Work out the finished part from the listing and answer in its coordinate system (mm). A direction names the side the tool comes from. Give positions to 0.01 mm unless a question says otherwise; leave off trailing zeros. Loops run counter-clockwise (first coordinate to the right, second up) from the corner with the lowest first, then second, coordinate; pieces in that order, holes last. Notation, with made-up numbers: M -33,-26.75 L 6,-26.75 A38 ccw 6,11.25 Z; hole C -2.5,-23 d9. An arc over 180 degrees is marked long. Write item = value, one per line. Start each with the question number.
1. Flat-ended cylindrical pins translate along their axes: pin 1 Ø2.5 at (x, y) = (-20.5, 6) entering from -Z; pin 2 Ø1.5 at (x, z) = (6, -4.5) entering from +Y; pin 3 Ø4 at (y, z) = (6.5, -16.5) entering from -X. Find the tip coordinate at first contact, or state that the pin passes through.
2. Section B-B on y = 6 is taken. Give the number of separate pieces and of enclosed holes in the cut face, plus the area to 3 significant figures.
3. For faces 1 (the face through (-21.89, 4.94, 20.07)), 2 (the face through (14, 8, -18)), 3 (the face through (24, 3, 6)), determine the directions among +Z, -Z, +X, -X, +Y, -Y from which every point of the face is accessible in a straight line to the end or side of a thin tool.
4. Section D-D on y = 1 is taken. Determine the outline of the cut face in (x, z), plus the area to 3 significant figures.
5. Consider L1, parallel to X at y = 2.4, z = -8.5; L2, parallel to X at y = 1.8, z = 9; L3, parallel to Y at x = -19.75, z = -17.5. Determine where each line is inside the solid, lowest interval first. Write a range as [from, to].
6. Section A-A on x = -20.5 is taken. Determine the outline of the cut face in (y, z), plus the area to 3 significant figures.
7. Section C-C on z = -17.5 is taken. Determine the outline of the cut face in (x, y), plus the area to 3 significant figures.
8. The mould has two halves that part along Z. Classify faces 4 (the face through (13.57, 2.03, -9.15)), 5 (the face through (-19.43, 2.03, -9.15)), 6 (the face through (-19, 6, -20.5)), 7 (the face through (-26, 2, 0)): released by +Z, released by -Z, zero draft, split by the parting line, or undercut.
```python
from build123d import *

# Parameters (mm, degrees)
SKETCH1_W               = 53
SKETCH1_H               = 55
TOP_DEPTH               = 2
SKETCH2_W               = 48
SKETCH2_H               = 50
INSIDE_LIP_DEPTH        = 2
SKETCH3_W               = 7
SKETCH3_H               = 10
SKETCH3_W_2             = 10
SKETCH3_H_2             = 6
SCREW_POSTS_DEPTH       = 5
SKETCH4_R               = 1.75
FRONT_SCREW_HOLES_DEPTH = 10
BACK_START              = -48
SKETCH5_R               = 1.6
BACK_SCREW_HOLES_DEPTH  = 48
SKETCH6_R               = 3
CUT_EXTRUDE3_DEPTH      = 4


with BuildPart() as part:
    # Sketch1 → Top (new body)
    with BuildSketch(Plane(origin=(0, 0, 0), x_dir=(1, 0, 0), z_dir=(0, 1, 0))):
        Rectangle(SKETCH1_W, SKETCH1_H)
    extrude(amount=TOP_DEPTH)

    # Sketch2 → Inside Lip (add)
    with BuildSketch(Plane(origin=(0, 2, 0), x_dir=(1, 0, 0), z_dir=(0, 1, 0))):
        Rectangle(SKETCH2_W, SKETCH2_H)
    extrude(amount=INSIDE_LIP_DEPTH)

    # Sketch3 → Screw Posts (add)
    with BuildSketch(Plane(origin=(0, 4, 0), x_dir=(1, 0, 0), z_dir=(0, 1, 0))):
        with Locations((-20.5, -20)):
            Rectangle(SKETCH3_W, SKETCH3_H)
        with Locations((20.5, -20)):
            Rectangle(SKETCH3_W, SKETCH3_H)
        with Locations((19, 17.5)):
            Rectangle(SKETCH3_W_2, SKETCH3_H_2)
        with Locations((-19, 17.5)):
            Rectangle(SKETCH3_W_2, SKETCH3_H_2)
    extrude(amount=SCREW_POSTS_DEPTH)

    # Sketch4 → Front Screw Holes (cut)
    with BuildSketch(Plane.XY.offset(25)):
        with Locations((-20.5, 6)):
            Circle(SKETCH4_R)
        with Locations((20.5, 6)):
            Circle(SKETCH4_R)
    extrude(amount=-FRONT_SCREW_HOLES_DEPTH, mode=Mode.SUBTRACT)

    # Sketch5 → Back Screw Holes (cut)
    with BuildSketch(Plane(origin=(24, 0, 0), x_dir=(0, 0, -1), z_dir=(1, 0, 0)).offset(BACK_START)):
        with Locations((17.5, 6)):
            Circle(SKETCH5_R)
    extrude(amount=BACK_SCREW_HOLES_DEPTH, mode=Mode.SUBTRACT)

    # Sketch6 → Cut-Extrude3 (cut)
    with BuildSketch(Plane(origin=(0, 4, 0), x_dir=(1, 0, 0), z_dir=(0, 1, 0))):
        with Locations(Location((-16.5, -9, 0), (0, 0, 270))):
            Circle(SKETCH6_R)
        with Locations(Location((-16.5, 8.5, 0), (0, 0, 270))):
            Circle(SKETCH6_R)
        with Locations(Location((16.5, -9, 0), (0, 0, 270))):
            Circle(SKETCH6_R)
        with Locations(Location((16.5, 8.5, 0), (0, 0, 270))):
            Circle(SKETCH6_R)
    extrude(amount=-CUT_EXTRUDE3_DEPTH, mode=Mode.SUBTRACT)


solid = part.part
```
Verdict:
q1.pin_1 = -20.5
q1.pin_2 = 4
q1.pin_3 = -24
q2.separate_pieces = 8
q2.enclosed_holes = 0
q2.area = 126 mm2
q3.face_1 = +Z
q3.face_2 = +Z, -Z, +Y
q3.face_3 = +Z, -Z, +X, +Y
q4.outline = M -26.5,-27.5 L 26.5,-27.5 L 26.5,27.5 L -26.5,27.5 Z; hole C -16.5,-8.5 d6; hole C -16.5,9 d6; hole C 16.5,-8.5 d6; hole C 16.5,9 d6
q4.area = 2,800 mm2
q5.L1 = [-24, -19.5], [-13.5, 13.5], [19.5, 24]
q5.L2 = [-26.5, -19.5], [-13.5, 13.5], [19.5, 26.5]
q5.L3 = [0, 4.4], [7.6, 9]
q6.outline = M 0,-27.5 L 2,-27.5 L 2,-25 L 4,-25 L 4,-20.5 L 9,-20.5 L 9,-14.5 L 4,-14.5 L 4,15 L 4.25,15 L 4.25,25 L 2,25 L 2,27.5 L 0,27.5 Z; M 7.75,15 L 9,15 L 9,25 L 7.75,25 Z; hole C 6,-17.5 d3.2
q6.area = 247 mm2
q7.outline = M -26.5,0 L 26.5,0 L 26.5,2 L 24,2 L 24,4.4 L 14,4.4 L 14,4 L -14,4 L -14,4.4 L -24,4.4 L -24,2 L -26.5,2 Z; M -24,7.6 L -14,7.6 L -14,9 L -24,9 Z; M 14,7.6 L 24,7.6 L 24,9 L 14,9 Z
q7.area = 238 mm2
q8.face_4 = undercut
q8.face_5 = undercut
q8.face_6 = released by -Z
q8.face_7 = zero draft
